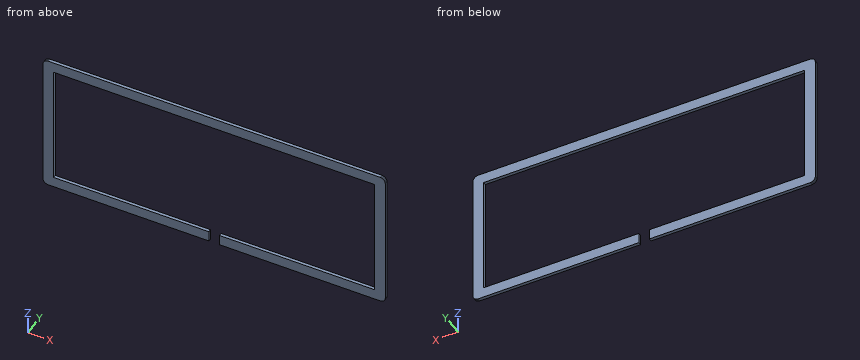
Autodesk Fusion 360 part; units mm, degrees
sketch "Sketch1" plane through (0, 0, 0) normal (0, 1, 0) x (1, 0, 0)
  line L0 (3.5485, 0.3183) -> (3.1805, 0.4548)
  line L1 (2.825, 0.6187) -> (2.4819, 0.8103)
  line L2 (2.1553, 1.028) -> (1.8466, 1.2706)
  line L3 (324.159, 131.987) -> (324.35, 131.644)
  line L4 (324.651, 130.92) -> (324.757, 130.542)
  line L5 (314.895, 10.0748) -> (314.895, 124.375)
  line L6 (321.441, 134.13) -> (321.809, 133.993)
  line L7 (3.1805, 0.4548) -> (2.825, 0.6187)
  line L8 (321.062, 134.236) -> (321.441, 134.13)
  line L9 (324.834, 130.157) -> (324.879, 129.767)
  line L10 (323.941, 2.1346) -> (323.698, 1.8259)
  line L11 (324.834, 4.2912) -> (324.757, 3.9067)
  line L12 (3.9274, 0.2122) -> (3.5485, 0.3183)
  line L13 (2.4819, 0.8103) -> (2.1553, 1.028)
  line L14 (167.495, 124.375) -> (167.495, 134.374)
  line L15 (1.5586, 1.5379) -> (1.2912, 1.8259)
  line L16 (321.062, 0.2122) -> (320.678, 0.135)
  line L17 (321.809, 0.4548) -> (321.441, 0.3183)
  line L18 (324.757, 3.9067) -> (324.651, 3.5278)
  line L19 (324.35, 2.8043) -> (324.159, 2.4612)
  line L20 (324.757, 130.542) -> (324.834, 130.157)
  line L21 (324.514, 131.288) -> (324.651, 130.92)
  line L22 (324.159, 2.4612) -> (323.941, 2.1346)
  line L23 (157.494, 124.375) -> (10.0941, 124.375)
  line L24 (323.431, 1.5379) -> (323.143, 1.2705)
  line L25 (157.494, 134.375) -> (157.494, 124.375)
  line L26 (320.678, 134.313) -> (321.062, 134.236)
  line L27 (323.431, 132.91) -> (323.698, 132.623)
  line L28 (324.879, 129.767) -> (324.895, 129.374)
  line L29 (10.0941, 10.0748) -> (314.895, 10.0748)
  line L30 (320.288, 0.0896) -> (319.896, 0.073)
  line L31 (319.896, 0.073) -> (5.0946, 0.073)
  line L32 (5.0946, 0.073) -> (4.7019, 0.0896)
  line L33 (0.6394, 131.644) -> (0.831, 131.987)
  line L34 (1.2912, 1.8259) -> (1.0487, 2.1346)
  line L35 (167.495, 134.374) -> (319.896, 134.374)
  line L36 (0.831, 2.4612) -> (0.6394, 2.8043)
  line L37 (1.8466, 1.2706) -> (1.5586, 1.5379)
  line L38 (323.941, 132.314) -> (324.159, 131.987)
  line L39 (10.0941, 124.375) -> (10.0941, 10.0748)
  line L40 (0.4754, 3.1598) -> (0.339, 3.5278)
  line L41 (322.508, 0.8103) -> (322.165, 0.6187)
  line L42 (0.0937, 5.0739) -> (0.0951, 129.374)
  line L43 (1.8466, 133.178) -> (2.1553, 133.42)
  line L44 (0.2329, 130.542) -> (0.339, 130.92)
  line L45 (3.1805, 133.993) -> (3.5485, 134.13)
  line L46 (323.698, 132.623) -> (323.941, 132.314)
  line L47 (324.895, 129.374) -> (324.896, 5.0726)
  line L48 (320.678, 0.135) -> (320.288, 0.0896)
  line L49 (324.35, 131.644) -> (324.514, 131.288)
  line L50 (322.834, 133.42) -> (323.143, 133.178)
  line L51 (0.0951, 129.374) -> (0.1102, 129.767)
  line L52 (3.5485, 134.13) -> (3.9274, 134.236)
  line L53 (0.1102, 4.6812) -> (0.0937, 5.0739)
  line L54 (5.0946, 134.375) -> (157.494, 134.375)
  line L55 (319.896, 134.374) -> (320.288, 134.359)
  line L56 (324.896, 5.0726) -> (324.879, 4.6812)
  line L57 (0.1557, 130.157) -> (0.2329, 130.542)
  line L58 (4.7019, 134.359) -> (5.0946, 134.375)
  line L59 (322.508, 133.638) -> (322.834, 133.42)
  line L60 (4.3119, 0.135) -> (3.9274, 0.2122)
  line L61 (324.514, 3.1598) -> (324.35, 2.8043)
  line L62 (4.7019, 0.0896) -> (4.3119, 0.135)
  line L63 (324.879, 4.6812) -> (324.834, 4.2912)
  line L64 (321.441, 0.3183) -> (321.062, 0.2122)
  line L65 (321.809, 133.993) -> (322.165, 133.829)
  line L66 (0.6394, 2.8043) -> (0.4754, 3.1598)
  line L67 (0.831, 131.987) -> (1.0487, 132.314)
  line L68 (0.339, 3.5278) -> (0.2329, 3.9067)
  line L69 (2.4819, 133.638) -> (2.825, 133.829)
  line L70 (1.2912, 132.623) -> (1.5586, 132.91)
  line L71 (322.834, 1.028) -> (322.508, 0.8103)
  line L72 (320.288, 134.359) -> (320.678, 134.313)
  line L73 (1.5586, 132.91) -> (1.8466, 133.178)
  line L74 (0.2329, 3.9067) -> (0.1557, 4.2912)
  line L75 (314.895, 124.375) -> (167.495, 124.375)
  line L76 (323.143, 1.2706) -> (322.834, 1.028)
  line L77 (324.651, 3.5278) -> (324.514, 3.1598)
  line L78 (0.339, 130.92) -> (0.4754, 131.288)
  line L79 (322.165, 0.6187) -> (321.809, 0.4548)
  line L80 (4.3119, 134.313) -> (4.7019, 134.359)
  line L81 (0.1557, 4.2912) -> (0.1102, 4.6812)
  line L82 (0.1102, 129.767) -> (0.1557, 130.157)
  line L83 (3.9274, 134.236) -> (4.3119, 134.313)
  line L84 (2.825, 133.829) -> (3.1805, 133.993)
  line L85 (323.698, 1.8259) -> (323.431, 1.5379)
  line L86 (2.1553, 133.42) -> (2.4819, 133.638)
  line L87 (1.0487, 2.1346) -> (0.831, 2.4612)
  line L88 (0.4754, 131.288) -> (0.6394, 131.644)
  line L89 (1.0487, 132.314) -> (1.2912, 132.623)
  line L90 (322.165, 133.829) -> (322.508, 133.638)
  line L91 (323.143, 133.178) -> (323.431, 132.91)
extrude "Extrude1" add sketch "Sketch1" along normal blind 3
Could you check a few things on this model? Use its own coordinates, in mm. Give positions to 0.01 mm unless a question says otherwise; leave off trailing zeros. Order: outer loops, then holes, each group sorted by start corner. A loop starts at its lowest first (then second) coordinate and runs counter-clockwise, first axis right, second up.
1. Suppose I cut it at B-B (z = -46). List the corners of the cut face in (x, y) for me (3 decimals), plus the area to 3 significant figures.
2. I need wall thicknesses on L1, parallel to X at y = 2.45, z = -110 (3 decimals); L2, parallel to Z at x = 124, y = 2.1 (3 decimals); L3, parallel to Z at x = 161, y = 0.35. Which ranges of each line are inside material? Lowest first, please.
3. Suppose I cut it at A-A (x = 55.5). List the corners of the cut face in (y, z) for me (3 decimals).
Solved:
1. outline: (0.094, 0) - (10.094, 0) - (10.094, 3) - (0.094, 3) - close; (314.895, 0) - (324.896, 0) - (324.896, 3) - (314.895, 3) - close
1. area: 60.0 mm2
2. L1: x = 0.095 to 10.094, 314.895 to 324.895
2. L2: z = -134.375 to -124.375, -10.075 to -0.073
2. L3: z = -10.07 to -0.07
3. outline: (0, -134.375) - (3, -134.375) - (3, -124.375) - (0, -124.375) - close; (0, -10.075) - (3, -10.075) - (3, -0.073) - (0, -0.073) - close
